Verification items for the finished model (mm, model axes). Face numbers are marked on the shaded views. A direction names the side the tool comes from. Give positions to 0.01 mm unless a question says otherwise; leave off trailing zeros. Loops run counter-clockwise (first coordinate to the right, second up) from the corner with the lowest first, then second, coordinate; pieces in that order, holes last. Notation, with made-up numbers: (-6.5, -14.75) - (40.5, -14.75) arc R32 ccw to (40.5, 21.25) - close; hole circle Ø5 at (75, 19.25). An arc over 180 degrees is marked (long way). Answer in a Markdown table with one row per item.
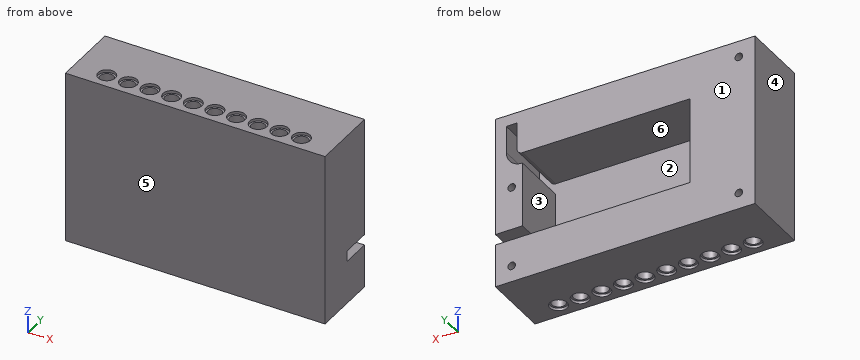
```python
from build123d import *

# Parameters (mm, degrees)
SKETCH1_W           = 96
SKETCH1_H           = 64
BOSS_EXTRUDE1_DEPTH = 4
BOSS_EXTRUDE2_DEPTH = 21
SKETCH3_W           = 10
SKETCH3_H           = 4
BOSS_EXTRUDE4_DEPTH = 10
SKETCH4_R           = 1.4
CUT_EXTRUDE1_DEPTH  = 20
SKETCH5_R           = 2.5
CUT_EXTRUDE2_DEPTH  = 10
SKETCH7_R           = 3.2
CUT_EXTRUDE3_DEPTH  = 1


with BuildPart() as part:
    # Sketch1 → Boss-Extrude1 (new body)
    with BuildSketch(Plane(origin=(0, 0, 0), x_dir=(1, 0, 0), z_dir=(0, 1, 0))):
        Rectangle(SKETCH1_W, SKETCH1_H)
    extrude(amount=BOSS_EXTRUDE1_DEPTH)

    # Sketch2 → Boss-Extrude2 (add)
    with BuildSketch(Plane(origin=(0, 4, 0), x_dir=(1, 0, 0), z_dir=(0, 1, 0))):
        with BuildLine():
            Line((38, 16), (48, 16))
            Line((48, 16), (48, 32))
            Line((48, 32), (-48, 32))
            Line((-48, 32), (-48, -32))
            Line((-48, -32), (48, -32))
            Line((48, -32), (48, 12))
            Line((48, 12), (38, 12))
            Line((38, 12), (38, -12))
            ThreePointArc((38, -12), (42.242640687, -13.757359313), (44, -18))
            Line((44, -18), (44, -28))
            Line((44, -28), (40, -28))
            Line((40, -28), (40, -18))
            ThreePointArc((40, -18), (39.414213562, -16.585786438), (38, -16))
            Line((38, -16), (-24, -16))
            Line((-24, -16), (-24, 16))
            Line((-24, 16), (38, 16))
        make_face()
    extrude(amount=BOSS_EXTRUDE2_DEPTH)

    # Sketch3 → Boss-Extrude4 (add)
    with BuildSketch(Plane(origin=(56, 4, -12), x_dir=(1, 0, 0), z_dir=(0, -1, 0))):
        with Locations((-13, -2)):
            Rectangle(SKETCH3_W, SKETCH3_H)
    extrude(amount=-BOSS_EXTRUDE4_DEPTH)

    # Sketch4 → Cut-Extrude1 (cut)
    with BuildSketch(Plane(origin=(0, 25, 0), x_dir=(1, 0, 0), z_dir=(0, 1, 0))):
        with Locations(Location((-42, 26, 0), (0, 0, 270))):
            Circle(SKETCH4_R)
        with Locations(Location((-42, -26, 0), (0, 0, 90))):
            Circle(SKETCH4_R)
        with Locations(Location((42, 26, 0), (0, 0, 90))):
            Circle(SKETCH4_R)
        with Locations(Location((42, -4, 0), (0, 0, 270))):
            Circle(SKETCH4_R)
    extrude(amount=-CUT_EXTRUDE1_DEPTH, mode=Mode.SUBTRACT)

    # Sketch5 → Cut-Extrude2 (cut)
    with BuildSketch(Plane.XY.offset(32)):
        with Locations((-36, 5.6)):
            Circle(SKETCH5_R)
        with Locations((-28, 5.6)):
            Circle(SKETCH5_R)
        with Locations((-20, 5.6)):
            Circle(SKETCH5_R)
        with Locations((-12, 5.6)):
            Circle(SKETCH5_R)
        with Locations((-4, 5.6)):
            Circle(SKETCH5_R)
        with Locations((4, 5.6)):
            Circle(SKETCH5_R)
        with Locations((12, 5.6)):
            Circle(SKETCH5_R)
        with Locations((20, 5.6)):
            Circle(SKETCH5_R)
        with Locations((28, 5.6)):
            Circle(SKETCH5_R)
        with Locations((36, 5.6)):
            Circle(SKETCH5_R)
    cut_extrude2 = extrude(amount=-CUT_EXTRUDE2_DEPTH, mode=Mode.SUBTRACT)

    # Sketch7 → Cut-Extrude3 (cut)
    with BuildSketch(Plane.XY.offset(32)):
        with Locations((-36, 5.6)):
            Circle(SKETCH7_R)
        with Locations((-28, 5.6)):
            Circle(SKETCH7_R)
        with Locations((-20, 5.6)):
            Circle(SKETCH7_R)
        with Locations((-12, 5.6)):
            Circle(SKETCH7_R)
        with Locations((-4, 5.6)):
            Circle(SKETCH7_R)
        with Locations((4, 5.6)):
            Circle(SKETCH7_R)
        with Locations((12, 5.6)):
            Circle(SKETCH7_R)
        with Locations((20, 5.6)):
            Circle(SKETCH7_R)
        with Locations((28, 5.6)):
            Circle(SKETCH7_R)
        with Locations((36, 5.6)):
            Circle(SKETCH7_R)
    cut_extrude3 = extrude(amount=-CUT_EXTRUDE3_DEPTH, mode=Mode.SUBTRACT)

    # Mirror1: Cut-Extrude2, Cut-Extrude3 across plane
    add(cut_extrude2.mirror(Plane.XY), mode=Mode.SUBTRACT)
    add(cut_extrude3.mirror(Plane.XY), mode=Mode.SUBTRACT)


solid = part.part
```
Q1. Sectioned sample at A-A (x = 20). Record the cut outline in (y, z), and give its area (3 significant figures).
Completed:
| item | result |
|---|---|
| outline | (0, -32) - (2.4, -32) - (2.4, -31) - (3.1, -31) - (3.1, -22) - (8.1, -22) - (8.1, -31) - (8.8, -31) - (8.8, -32) - (25, -32) - (25, -16) - (4, -16) - (4, 16) - (25, 16) - (25, 32) - (8.8, 32) - (8.8, 31) - (8.1, 31) - (8.1, 22) - (3.1, 22) - (3.1, 31) - (2.4, 31) - (2.4, 32) - (0, 32) - close |
| area | 825 mm^2 |
Q2. Go/stop test with flat-tipped pins: P1, Ø1.5, axis at x = -12.5, y = 5, coming from the -Z side; P2, Ø1.5, axis at x = -5, y = 5.5, coming from the +Z side; P3, Ø3, axis at x = 28.5, y = 4.5, coming from the -Z side. Record where each tip stops, or that it passes through.
Completed:
| item | result |
|---|---|
| P1 | z = -22 |
| P2 | z = 22 |
| P3 | z = -31 |
Q3. Sectioned sample at B-B (y = 10.75). Record the cut outline in (x, z), and give its area (3 significant figures).
Completed:
| item | result |
|---|---|
| outline | (-48, -32) - (48, -32) - (48, 32) - (-48, 32) - close; hole circle Ø2.8 at (-42, -26); hole circle Ø2.8 at (-42, 26); hole (-24, -16) - (38, -16) - (38, 12) arc R6 ccw to (44, 18) - (44, 28) - (40, 28) - (40, 18) arc R2 cw to (38, 16) - (-24, 16) - close; hole circle Ø2.8 at (42, -26); hole circle Ø2.8 at (42, 4) |
| area | 4,070 mm^2 |
Q4. Sectioned sample at C-C (z = -26). Give the number of separate pieces and of enclosed holes in the cut face, and give its area (3 significant figures).
Completed:
| item | result |
|---|---|
| separate pieces | 1 |
| enclosed holes | 10 |
| area | 2,090 mm^2 |
Q5. Sectioned sample at D-D (y = 17). Record the cut outline in (x, z).
Completed:
| item | result |
|---|---|
| outline | (-48, -32) - (48, -32) - (48, -16) - (-24, -16) - (-24, 16) - (38, 16) arc R2 ccw to (40, 18) - (40, 28) - (44, 28) - (44, 18) arc R6 cw to (38, 12) - (38, -12) - (48, -12) - (48, 32) - (-48, 32) - close; hole circle Ø2.8 at (-42, -26); hole circle Ø2.8 at (-42, 26); hole circle Ø2.8 at (42, -26); hole circle Ø2.8 at (42, 4) |
Q6. Thickness scan on line 1 (X direction, y = 15, z = -26); line 2 (X direction, y = 19.25, z = -9); line 3 (Z direction, x = 28, y = 22.75). Record the ranges inside material, lowest first.
Completed:
| item | result |
|---|---|
| line 1 | -48 to -43.4, -40.6 to 40.6, 43.4 to 48 |
| line 2 | -48 to -24, 38 to 48 |
| line 3 | -32 to -16, 16 to 32 |
Q7. Draft check along X on the marked faces 1, 2, 3 and 4. Enter one of: +X half, -X half, draft (parallel to the pull), parting line (faces both ways), or undercut.
Completed:
| item | result |
|---|---|
| face 1 | draft |
| face 2 | undercut |
| face 3 | undercut |
| face 4 | -X half |
Q8. Tool access check on the marked faces 5 and 6. Record the directions out of +Z, -Z, +X, -X, +Y, -Y that give a thin tool (end or side, any length) a straight path to the whole face; none if there is none.
Completed:
| item | result |
|---|---|
| face 5 | +Z, -Z, +X, -X, -Y |
| face 6 | +Y |
